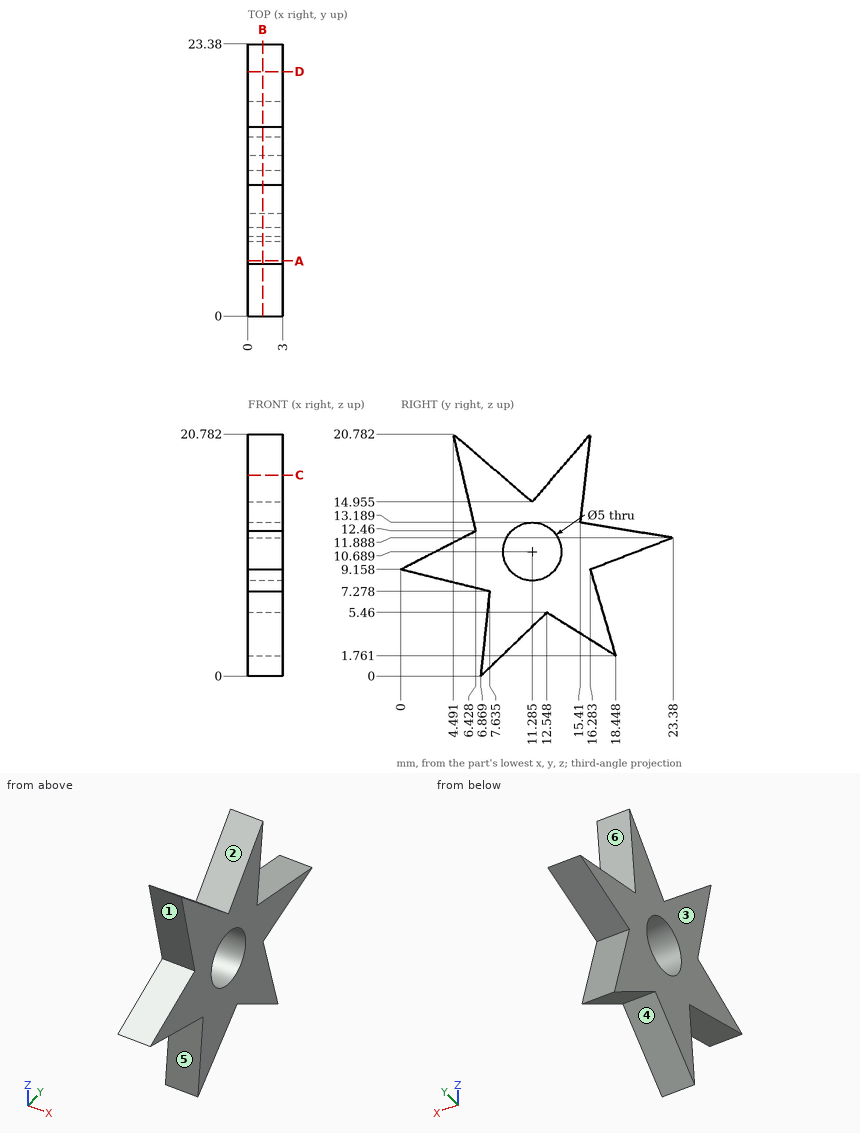
Verification items for this drawing (mm, ordinates from the low corner). A direction names the side the tool comes from. Coordinates: 2 decimals unless noted, no trailing zeros. Order: outer loops, then holes, each group sorted by start corner. A loop starts at its lowest first (then second) coordinate and runs counter-clockwise, first axis right, second up. Notation, with made-up numbers: M 77.25,79 L 95.25,79 A25 cw 95.25,97 Z; hole C 77.25,-35.5 d6. An arc over 180 degrees is marked long. Write each question's results on one line, items separated by ' | '.
1) Access from +Z, -Z, +X, -X, +Y, -Y to the whole of each face (thin tool, end or side, straight path). Record for the marked faces 4, 5 and 6.
Solved:
face 4: -Z, +X, -X | face 5: +X, -X, -Y | face 6: +X, -X, +Y
2) Section check D-D on y = 21. Record the cut outline in (x, z).
Solved:
outline: M 0,10.97 L 3,10.97 L 3,12.28 L 0,12.28 Z
3) Section check A-A on y = 4.75. Record the cut outline in (x, z).
Solved:
outline: M 0,7.99 L 3,7.99 L 3,11.6 L 0,11.6 Z; M 0,19.67 L 3,19.67 L 3,20.56 L 0,20.56 Z
4) Section check B-B on x = 1.25. Record the cut outline in (y, z) (1 decimal), plus the area to 3 significant figures.
Solved:
outline: M 0,9.2 L 7.6,7.3 L 6.9,0 L 12.5,5.5 L 18.4,1.8 L 16.3,9.2 L 23.4,11.9 L 15.4,13.2 L 16.3,20.8 L 11.3,15 L 4.5,20.8 L 6.4,12.5 Z; hole C 11.3,10.7 d5 | area: 154 mm²
5) Release check for a two-part mould opening along Z. For the marked faces 1, 2 and 3 record: pulls with the +Z half, pulls with the -Z half, needs draft (parallel to the pull), parting line crosses it, or undercut.
Solved:
face 1: undercut | face 2: pulls with the +Z half | face 3: needs draft
6) Scan lines: line 1 along Y through (x, z) = (2.1, 16.5) (1 decimal); line 2 along Y through (x, z) = (1.3, 6.75); line 3 along Z through (x, y) = (0.2, 8.75). Record each from-to range of solid material in increasing order. Write a range as [from, to].
Solved:
line 1: y = [5.5, 9.5], [12.6, 15.8] | line 2: y = [7.58, 16.99] | line 3: z = [1.81, 17.13]
7) Section check C-C on z = 17.25. Record the cut outline in (x, y).
Solved:
outline: M 0,5.31 L 3,5.31 L 3,8.61 L 0,8.61 Z; M 0,13.25 L 3,13.25 L 3,15.88 L 0,15.88 Z
